from build123d import *

# Parameters (mm, degrees)
EXTRUDE1_DEPTH               = 150
SHEET_METAL_1_DEPTH          = 150
SHEET_METAL_1_2_DEPTH        = 150
EDGE_FLANGE1_STRIP_W         = 6.5
EDGE_FLANGE1_STRIP_H         = 1
EDGE_FLANGE1_STRIP_CUT_DEPTH = 235.5
EDGE_FLANGE1_DEPTH           = 235.5
SKETCH16_W                   = 1
SKETCH16_H                   = 32.75
EXTRUDE2_DEPTH               = 2.25
EDGE_FLANGE2_DEPTH           = 235.5
EDGE_FLANGE2_START           = 1
EDGE_FLANGE2_FLAT_DEPTH      = 1


# Read off the part's stored shape, not the designer's step: Преобразовать-Твердое тело1
# Sheet-metal steps are written as plain solids
with BuildPart() as part:
    # Sketch1 → Extrude1 (new body)
    with BuildSketch(Plane.XY):
        Polygon((-120, 0), (-120, 35), (120, 35), (120, 0), (119, 0), (119, 34), (-119, 34), (-119, 0), align=None)
    extrude(amount=EXTRUDE1_DEPTH)

    # Sheet Metal 1 outline → Sheet Metal 1 (cut)
    with BuildSketch(Plane.XY):
        with BuildLine():
            Line((120, 35), (117.75, 35))
            ThreePointArc((117.75, 35), (119.340990258, 34.340990258), (120, 32.75))
            Line((120, 32.75), (120, 35))
        make_face()
        with BuildLine():
            ThreePointArc((-120, 32.75), (-119.340990258, 34.340990258), (-117.75, 35))
            Line((-117.75, 35), (-120, 35))
            Line((-120, 35), (-120, 32.75))
        make_face()
    extrude(amount=SHEET_METAL_1_DEPTH, mode=Mode.SUBTRACT)

    # Sheet Metal 1 2 outline → Sheet Metal 1 2 (add)
    with BuildSketch(Plane.XY):
        with BuildLine():
            Line((119, 34), (117.75, 34))
            ThreePointArc((117.75, 34), (118.633883476, 33.633883476), (119, 32.75))
            Line((119, 32.75), (119, 34))
        make_face()
        with BuildLine():
            ThreePointArc((-119, 32.75), (-118.633883476, 33.633883476), (-117.75, 34))
            Line((-117.75, 34), (-119, 34))
            Line((-119, 34), (-119, 32.75))
        make_face()
    extrude(amount=SHEET_METAL_1_2_DEPTH)

    # Edge-Flange1 strip (across the edge) → Edge-Flange1 strip cut (cut)
    with BuildSketch(Plane(origin=(117.75, 35, 0), x_dir=(0, 0, 1), z_dir=(-1, 0, 0))):
        with Locations((-1, -0.5)):
            Rectangle(EDGE_FLANGE1_STRIP_W, EDGE_FLANGE1_STRIP_H)
    extrude(amount=EDGE_FLANGE1_STRIP_CUT_DEPTH, mode=Mode.SUBTRACT)

    # Edge-Flange1 section (across the edge) → Edge-Flange1 (add)
    with BuildSketch(Plane(origin=(117.75, 35, 0), x_dir=(0, 0, 1), z_dir=(-1, 0, 0))):
        with BuildLine():
            Line((0, 1.25), (0, 11))
            Line((0, 11), (1, 11))
            Line((1, 11), (1, 1.25))
            ThreePointArc((1, 1.25), (1.366116524, 0.366116524), (2.25, 0))
            Line((2.25, 0), (2.25, -1))
            ThreePointArc((2.25, -1), (0.659009742, -0.340990258), (0, 1.25))
        make_face()
    extrude(amount=EDGE_FLANGE1_DEPTH)

    # Sketch16 → Extrude2 (add)
    with BuildSketch(Plane.XY.offset(150)):
        with Locations((-119.5, 16.375)):
            Rectangle(SKETCH16_W, SKETCH16_H)
        with Locations((119.5, 16.375)):
            Rectangle(SKETCH16_W, SKETCH16_H)
    extrude(amount=EXTRUDE2_DEPTH)

    # Edge-Flange2 bend section (across the edge) → Edge-Flange2 (add)
    with BuildSketch(Plane(origin=(117.75, 34, 151.25), x_dir=(0, 0, -1), z_dir=(-1, 0, 0))):
        with BuildLine():
            Line((-1, 1.25), (0, 1.25))
            ThreePointArc((0, 1.25), (0.366116524, 0.366116524), (1.25, 0))
            Line((1.25, 0), (1.25, -1))
            ThreePointArc((1.25, -1), (-0.340990258, -0.340990258), (-1, 1.25))
        make_face()
    extrude(amount=EDGE_FLANGE2_DEPTH)

    # Edge-Flange2 profile (on flange) → Edge-Flange2 flat (add)
    with BuildSketch(Plane(origin=(0, 34, 151.25), x_dir=(-1, 0, 0), z_dir=(0, 0, 1)).offset(EDGE_FLANGE2_START)):
        Polygon((-117.75, 1.35), (-117.75, 1.25), (117.75, 1.25), (117.75, 1.5), (118.8, 1.5), (118.8, 34), (-118.8, 34), (-118.8, 1.35), align=None)
    extrude(amount=-EDGE_FLANGE2_FLAT_DEPTH)


solid = part.part
Geometry check sheet. Reference: the model listing, model coordinates, mm. A direction names the side the tool comes from. Give positions to 0.01 mm unless a question says otherwise; leave off trailing zeros. Loops run counter-clockwise (first coordinate to the right, second up) from the corner with the lowest first, then second, coordinate; pieces in that order, holes last. Notation, with made-up numbers: M 49,43 L 58,43 A16 ccw 58,58 Z; hole C 81,72 d3. An arc over 180 degrees is marked long. Answer as a JSON object with one key per item and string values. Group by question number.
Item 1: Sectioned sample at C-C on z = 62.5. Record the boundary of the cut face in (x, y), plus the area to 3 significant figures.
Item 2: Material ranges on L1, parallel to X at y = 2.5, z = 115; L2, parallel to Y at x = 102.5, z = 68.5; L3, parallel to Z at x = -80.5, y = 21, recorded low to high.
Item 3: Sectioned sample at D-D on y = 39.5. Record the boundary of the cut face in (x, z), plus the area to 4 significant figures.
Item 4: Sectioned sample at B-B on x = -76. Record the boundary of the cut face in (y, z), plus the area to 3 significant figures.
Item 5: Mould release check, pull along X, two halves, no side actions. Record for faces 1 (the flat face through (-120, 16, 75)), 2 (the flat face through (2, 41, 0)), 3 (the flat face through (119, 16, 75)): pulls with the +X half, pulls with the -X half, needs draft (parallel to the pull), parting line crosses it, or undercut.
Item 6: Access from +Z, -Z, +X, -X, +Y, -Y to the whole of each face (thin tool, end or side, straight path). Record for faces 4 (the flat face through (-119, 16, 75)), 5 (the flat face through (2, 34, 75)), 6 (the flat face through (2, 16, 152.25)), 7 (the flat face through (120, 17, 75)), 8 (the flat face through (2, 41, 1)).
Item 7: Sectioned sample at A-A on y = 17. Record the boundary of the cut face in (x, z).
Item 8: Gauge pin test, flat ends, axial feed: pin 1 (5 mm diameter, centred on x = -6.5, y = 39.5, fed in from +Z); pin 2 (0.8 mm diameter, centred on x = 118.5, z = 151.5, fed in from +Y); pin 3 (12 mm diameter, centred on x = 72.5, y = 41.5, fed in from +Z); pin 4 (1 mm diameter, centred on y = 36, z = 67.5, fed in from +X). Record the tip position at first contact, or that the pin passes through.
Findings below:
{
 "1": {"outline": "M -120,0 L -119,0 L -119,32.75 A1.25 cw -117.75,34 L 117.75,34 A1.25 cw 119,32.75 L 119,0 L 120,0 L 120,32.75 A2.25 ccw 117.75,35 L -117.75,35 A2.25 ccw -120,32.75 Z", "area": "306 mm2"},
 "2": {"L1": "-120 to -119, 119 to 120", "L2": "34 to 35", "L3": "151.25 to 152.25"},
 "3": {"outline": "M -117.75,0 L 117.75,0 L 117.75,1 L -117.75,1 Z", "area": "235.5 mm2"},
 "4": {"outline": "M 0,151.25 L 32.75,151.25 A1.25 cw 34,150 L 34,2.25 A2.25 ccw 36.25,0 L 46,0 L 46,1 L 36.25,1 A1.25 cw 35,2.25 L 35,150 A2.25 ccw 32.75,152.25 L 0,152.25 Z", "area": "196 mm2"},
 "5": {"face 1": "pulls with the -X half", "face 2": "needs draft", "face 3": "undercut"},
 "6": {"face 4": "+Z, -Z, -Y", "face 5": "-Z, -Y", "face 6": "+Z, +X, -X, +Y, -Y", "face 7": "+Z, -Z, +X, +Y, -Y", "face 8": "+Z, +X, -X, +Y"},
 "7": {"outline": "M -120,0 L -119,0 L -119,152.25 L -120,152.25 Z; M -118.8,151.25 L 118.8,151.25 L 118.8,152.25 L -118.8,152.25 Z; M 119,0 L 120,0 L 120,152.25 L 119,152.25 Z"},
 "8": {"pin 1": "z = 1", "pin 2": "y = 32.65", "pin 3": "z = 1.25", "pin 4": "through"}
}
